Check sheet for the modelled part. Datum: model origin and axes. Units: mm. Coordinates: 2 decimals unless noted, no trailing zeros. Order: outer loops, then holes, each group sorted by start corner. A loop starts at its lowest first (then second) coordinate and runs counter-clockwise, first axis right, second up. Notation, with made-up numbers: (22, -11.5) -> (64, -11.5) arc R16 ccw to (64, 19.5) -> close; hole circle Ø3 at (39.25, 58.25). An arc over 180 degrees is marked (long way). Put each result on its own line as item: value. Start each with the question number.
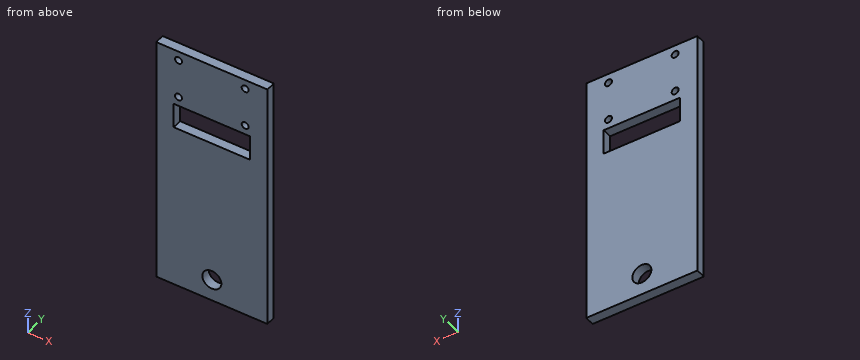
```python
from build123d import *

# Parameters (mm, degrees)
SKETCH1_W           = 35
SKETCH1_H           = 80
SKETCH1_R           = 1.1
BOSS_EXTRUDE1_DEPTH = 3
SKETCH2_R           = 3
CUT_EXTRUDE1_DEPTH  = 4
SKETCH3_W           = 24
SKETCH3_H           = 8
CUT_EXTRUDE2_DEPTH  = 4


with BuildPart() as part:
    # Sketch1 → Boss-Extrude1 (new body)
    with BuildSketch(Plane(origin=(0, 0, 0), x_dir=(1, 0, 0), z_dir=(0, 1, 0))):
        with Locations((17.5, 40)):
            Rectangle(SKETCH1_W, SKETCH1_H)
        with Locations((7, 3)):
            Circle(SKETCH1_R, mode=Mode.SUBTRACT)
        with Locations((28, 3)):
            Circle(SKETCH1_R, mode=Mode.SUBTRACT)
        with Locations((7, 15.5)):
            Circle(SKETCH1_R, mode=Mode.SUBTRACT)
        with Locations((28, 15.5)):
            Circle(SKETCH1_R, mode=Mode.SUBTRACT)
    extrude(amount=BOSS_EXTRUDE1_DEPTH)

    # Sketch2 → Cut-Extrude1 (cut, through all)
    with BuildSketch(Plane.XZ):
        with Locations((17.5, -73)):
            Circle(SKETCH2_R)
    extrude(amount=-CUT_EXTRUDE1_DEPTH, mode=Mode.SUBTRACT)

    # Sketch3 → Cut-Extrude2 (cut, through all)
    with BuildSketch(Plane(origin=(0, 3, 0), x_dir=(1, 0, 0), z_dir=(0, 1, 0))):
        with Locations((17.5, 22.5)):
            Rectangle(SKETCH3_W, SKETCH3_H)
    extrude(amount=-CUT_EXTRUDE2_DEPTH, mode=Mode.SUBTRACT)


solid = part.part
```
1) Sectioned sample at D-D (z = -3). Record the boundary of the cut face in (x, y).
2) Sectioned sample at A-A (z = -22). Record the boundary of the cut face in (x, y).
3) Sectioned sample at B-B (y = 1.25). Record the boundary of the cut face in (x, z).
4) Scan lines: line 1 along Z through (x, y) = (7, 1.2); line 2 along Z through (x, y) = (23.5, 1.9); line 3 along X through (y, z) = (0.5, -21). Record each from-to range of solid material in increasing order. Write a range as [from, to].
5) Sectioned sample at C-C (x = 7). Record the boundary of the cut face in (y, z).
Entries:
1. outline: (0, 0) -> (5.9, 0) -> (5.9, 3) -> (0, 3) -> close; (8.1, 0) -> (26.9, 0) -> (26.9, 3) -> (8.1, 3) -> close; (29.1, 0) -> (35, 0) -> (35, 3) -> (29.1, 3) -> close
2. outline: (0, 0) -> (5.5, 0) -> (5.5, 3) -> (0, 3) -> close; (29.5, 0) -> (35, 0) -> (35, 3) -> (29.5, 3) -> close
3. outline: (0, -80) -> (35, -80) -> (35, 0) -> (0, 0) -> close; hole (5.5, -26.5) -> (29.5, -26.5) -> (29.5, -18.5) -> (5.5, -18.5) -> close; hole circle Ø2.2 at (7, -15.5); hole circle Ø2.2 at (7, -3); hole circle Ø6 at (17.5, -73); hole circle Ø2.2 at (28, -15.5); hole circle Ø2.2 at (28, -3)
4. line 1: z = [-80, -26.5], [-18.5, -16.6], [-14.4, -4.1], [-1.9, 0]
4. line 2: z = [-80, -26.5], [-18.5, 0]
4. line 3: x = [0, 5.5], [29.5, 35]
5. outline: (0, -80) -> (3, -80) -> (3, -26.5) -> (0, -26.5) -> close; (0, -18.5) -> (3, -18.5) -> (3, -16.6) -> (0, -16.6) -> close; (0, -14.4) -> (3, -14.4) -> (3, -4.1) -> (0, -4.1) -> close; (0, -1.9) -> (3, -1.9) -> (3, 0) -> (0, 0) -> close
